```python
from build123d import *

# Parameters (mm, degrees)
F0_R     = 3.175
F0_R_2   = 25
F1_DEPTH = 1.5
F2_R     = 20


with BuildPart() as f1:
    # F0 (on Front) → F1 (new body)
    with BuildSketch(Plane.XZ):
        with BuildLine():
            Line((-17.829632, -30.118171), (-8.660254, -46))
            ThreePointArc((-8.660254, -46), (0, -51), (8.660254, -46))
            Line((8.660254, -46), (17.829632, -30.118171))
            ThreePointArc((17.829632, -30.118171), (30.310889, -17.5), (34.997917, -0.381829))
            Line((34.997917, -0.381829), (44.167296, 15.5))
            ThreePointArc((44.167296, 15.5), (44.167296, 25.5), (35.507042, 30.5))
            Line((35.507042, 30.5), (17.168285, 30.5))
            ThreePointArc((17.168285, 30.5), (0, 35), (-17.168285, 30.5))
            Line((-17.168285, 30.5), (-35.507042, 30.5))
            ThreePointArc((-35.507042, 30.5), (-44.167296, 25.5), (-44.167296, 15.5))
            Line((-44.167296, 15.5), (-34.997917, -0.381829))
            ThreePointArc((-34.997917, -0.381829), (-30.310889, -17.5), (-17.829632, -30.118171))
        make_face()
        with Locations((0, -41)):
            Circle(F0_R, mode=Mode.SUBTRACT)
        with Locations((-35.507042, 20.5)):
            Circle(F0_R, mode=Mode.SUBTRACT)
        Circle(F0_R_2, mode=Mode.SUBTRACT)
        with Locations((35.507042, 20.5)):
            Circle(F0_R, mode=Mode.SUBTRACT)
    extrude(amount=F1_DEPTH)

    # F2
    f2_edges = [f1.edges().sort_by_distance(p)[0] for p in [
        (34.997917, -0.75, -0.381829),
        (17.168285, -0.75, 30.5),
        (-17.168285, -0.75, 30.5),
        (-34.997917, -0.75, -0.381829),
        (-17.829632, -0.75, -30.118171),
        (17.829632, -0.75, -30.118171),
    ]]
    fillet(f2_edges, radius=F2_R)


solid = f1.part
```
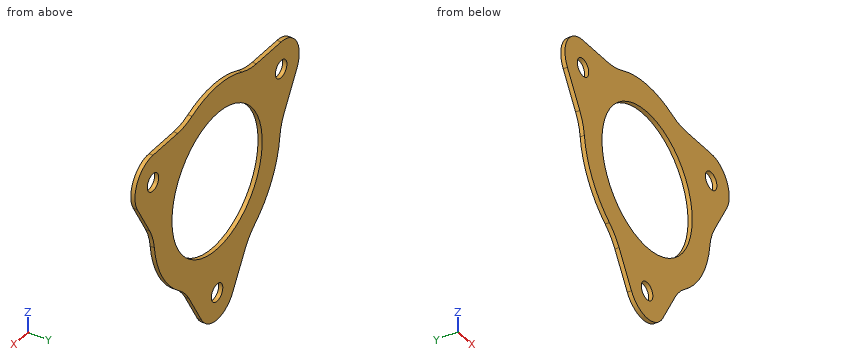
Could you check a few things on this model? Use its own coordinates, in mm. Coordinates: 2 decimals unless noted, no trailing zeros. Write each loop counter-clockwise with the first axis right and the second up, starting at its lowest first coordinate (ties: lowest second). Pieces come first, ordered by that corner, then holes. Notation, with made-up numbers: (4, 82) -> (48, 82) arc R33 cw to (48, 114) -> close; hole circle Ø3 at (24, -39.75). An arc over 180 degrees is marked (long way). Write item = value, one per line. Start each with the question number.
(1) I want a section at B-B (z = 20.5). Please give me the cut outline in (x, y), plus the area to 3 significant figures.
(2) I want a section at A-A (x = 0). Please give me the cut outline in (y, z) (3 decimals).
(3) I need wall thicknesses on line 1 (X direction, y = -1.15, z = 20); line 2 (X direction, y = -0.1, z = -16.5); line 3 (Z direction, x = -14, y = -0.9). Which ranges of each line are inside material? Lowest first, please. Write a range as [from, to].
(4) Will this pin go through, and if not, where does the flat tip stop? pin 1 (5.5 mm diameter, centred on x = -35.51, z = 20.5, fed in from +Y).
(5) I want a section at C-C (y = -0.6). Please give me the cut outline in (x, z) (3 decimals).
(6) I want a section at D-D (z = 2.5). Please give me the cut outline in (x, y), plus the area to 3 significant figures.
Result set:
q1.outline = (-45.51, -1.5) -> (-38.68, -1.5) -> (-38.68, 0) -> (-45.51, 0) -> close; (-32.33, -1.5) -> (-14.31, -1.5) -> (-14.31, 0) -> (-32.33, 0) -> close; (14.31, -1.5) -> (32.33, -1.5) -> (32.33, 0) -> (14.31, 0) -> close; (38.68, -1.5) -> (45.51, -1.5) -> (45.51, 0) -> (38.68, 0) -> close
q1.area = 74.5 mm2
q2.outline = (-1.5, -51) -> (0, -51) -> (0, -44.175) -> (-1.5, -44.175) -> close; (-1.5, -37.825) -> (0, -37.825) -> (0, -25) -> (-1.5, -25) -> close; (-1.5, 25) -> (0, 25) -> (0, 35) -> (-1.5, 35) -> close
q3.line_1 = [-45.49, -38.64], [-32.37, -15], [15, 32.37], [38.64, 45.49]
q3.line_2 = [-30.87, -18.78], [18.78, 30.87]
q3.line_3 = [-36.75, -20.71], [20.71, 32.08]
q4.pin_1 = through
q5.outline = (-44.167, 15.5) -> (-37.308, 3.62) arc R20 cw to (-34.764, -4.06) arc R35 ccw to (-20.898, -28.076) arc R20 cw to (-15.519, -34.12) -> (-8.66, -46) arc R10 ccw to (8.66, -46) -> (15.519, -34.12) arc R20 cw to (20.898, -28.076) arc R35 ccw to (34.764, -4.06) arc R20 cw to (37.308, 3.62) -> (44.167, 15.5) arc R10 ccw to (35.507, 30.5) -> (21.789, 30.5) arc R20 cw to (13.866, 32.136) arc R35 ccw to (-13.866, 32.136) arc R20 cw to (-21.789, 30.5) -> (-35.507, 30.5) arc R10 ccw to start; hole circle Ø6.35 at (-35.507, 20.5); hole circle Ø50 at (0, 0); hole circle Ø6.35 at (0, -41); hole circle Ø6.35 at (35.507, 20.5)
q6.outline = (-36.71, -1.5) -> (-24.87, -1.5) -> (-24.87, 0) -> (-36.71, 0) -> close; (24.87, -1.5) -> (36.71, -1.5) -> (36.71, 0) -> (24.87, 0) -> close
q6.area = 35.5 mm2
